```python
from build123d import *

# Parameters (mm, degrees)
F0_W     = 200
F0_H     = 250
F1_DEPTH = 8
F3_D     = 12


with BuildPart() as f1:
    # F0 (on Top) → F1 (new body)
    with BuildSketch(Plane.XY):
        with Locations((100, 125)):
            Rectangle(F0_W, F0_H)
    extrude(amount=F1_DEPTH)

    # F3 (through all)
    with Locations(Plane.XY.offset(8)):
        with Locations((25, 225), (25, 25), (175, 225), (175, 225), (175, 25)):
            Hole(F3_D / 2)


solid = f1.part
```
Here's how the part is built. I have some questions about the finished solid (model axes, mm). Coordinates: 2 decimals unless noted, no trailing zeros. Loops run counter-clockwise (first coordinate to the right, second up) from the corner with the lowest first, then second, coordinate; pieces in that order, holes last. Notation, with made-up numbers: (6.25, -17) - (17.25, -17) arc R27 ccw to (17.25, 5) - close; hole circle Ø2 at (74, 7). An arc over 180 degrees is marked (long way). Answer as CSV lines item,"result".
Q1. If we section it at A-A, the plane y = 225: Write out the boundary of the cut face in (x, z).
Response:
outline,"(0, 0) - (19, 0) - (19, 8) - (0, 8) - close; (31, 0) - (169, 0) - (169, 8) - (31, 8) - close; (181, 0) - (200, 0) - (200, 8) - (181, 8) - close"
Q2. If I drill on L1, parallel to Y at x = 25, z = 4.75; L2, parallel to X at y = 27, z = 6.5; L3, parallel to Y at x = 176.5, z = 6.25, over which ranges is the centre line in solid material (lowest first)? Write a range as [from, to].
Response:
L1,"[0, 19], [31, 219], [231, 250]"
L2,"[0, 19.34], [30.66, 169.34], [180.66, 200]"
L3,"[0, 19.19], [30.81, 219.19], [230.81, 250]"
Q3. For pin 1 (3 mm diameter, centred on x = 162.5, z = 3, fed in from -Y), with a flat end and sliding along its axis, tell me the tip position at first contact or that it passes through.
Response:
pin 1,"y = 0"
Q4. If we section it at B-B, the plane x = 25: Write out the boundary of the cut face in (y, z).
Response:
outline,"(0, 0) - (19, 0) - (19, 8) - (0, 8) - close; (31, 0) - (219, 0) - (219, 8) - (31, 8) - close; (231, 0) - (250, 0) - (250, 8) - (231, 8) - close"
Q5. We'd pull the mould along Y, two halves only. Please class faces 1 (the face through (99, 250, 4)), 2 (the face through (99, 127, 0)), 3 (the face through (29.76, 21.35, 3.94)): pulls with the +Y half, pulls with the -Y half, needs draft (parallel to the pull), parting line crosses it, or undercut.
Response:
face 1,"pulls with the +Y half"
face 2,"needs draft"
face 3,"undercut"
